Design review of the part built by this model. Coordinates are the model's own, in mm. A direction names the side the tool comes from. Coordinates: 2 decimals unless noted, no trailing zeros. Write each loop counter-clockwise with the first axis right and the second up, starting at its lowest first coordinate (ties: lowest second). Pieces come first, ordered by that corner, then holes.
Q1. Clearance check with flat-ended pins moving along their axes: pin 1 Ø1 at (x, z) = (-9.5, 1.5) entering from -Y; pin 2 Ø8 at (x, y) = (8, 9) entering from -Z; pin 3 Ø3.5 at (x, y) = (0, 6.25) entering from +Z; pin 4 Ø5 at (x, y) = (0, 6.35) entering from -Z. State where each tip first meets the part, or that it passes through.
Q2. Add section A-A, the plane x = 0. Give the boundary of the cut face in (y, z), plus the area to 3 significant figures.
Q3. Add section B-B, the plane z = -9.5. Give the boundary of the cut face in (x, y).
Q4. The part is to be moulded in two halves that separate along X. For faces 1 (the face through (0, 16, 0)), 2 (the face through (-0.9, 7.98, -6.2)), 3 (the face through (-1.009, 9.666, -15.267)), say which applies: +X half, -X half, draft (parallel to the pull), parting line (faces both ways), or undercut.
Q5. To check wall thickness, follow probe 1 along Y at (x, z) = (0, -6.3); probe 2 along X at (y, z) = (7.5, -7); probe 3 along X at (y, z) = (6.35, 12.5). State the ranges of each line that lie inside material, in increasing order.
Q6. Add section C-C, the plane z = 0. Give the boundary of the cut face in (x, y), plus the area to 3 significant figures.
Q7. Machinability: for faces 4 (the face through (-0.931, 3.393, 12.005)), 5 (the face through (-3, 0, 4)), 6 (the face through (0.931, 3.393, -12.005)), 7 (the face through (-4.34, 6.41, 1.8)), which of the approach directions +Z, -Z, +X, -X, +Y, -Y give a long, thin tool a straight path to every point of the face, cutting with its end or side? Answer none if there is none.
Q8. Add section D-D, the plane y = 13.5. Give the boundary of the cut face in (x, z).
Autodesk Inventor part; units mm, degrees
ref_plane "YZ Plane" through (0, 0, 0) normal (1, 0, 0) x (0, 1, 0)
ref_plane "XZ Plane" through (0, 0, 0) normal (0, 1, 0) x (-1, 0, 0)
ref_plane "XY Plane" through (0, 0, 0) normal (0, 0, 1) x (1, 0, 0)
sketch "Sketch1" plane through (0, 0, 0) normal (0, 1, 0) x (-1, 0, 0)
  circle A0 centre (0, 0) radius 15.3
  circle A1 centre (0, 0) radius 4.7
  dimension "d0" = 30.6
  dimension "d1" = 9.4
extrude "Extrusion1" add sketch "Sketch1" along normal blind 13
sketch "Sketch2" plane through (0, 13, 0) normal (0, 1, 0) x (1, 0, 0)
  line L0 (19.8933, 0) -> (-23.0575, 0) construction
  point P0 (0, 0)
ref_plane "Work Plane1" through (19.8933, 13, 0) normal (0, 0, -1) x (-1, 0, 0)
sketch "Sketch3" plane through (19.8933, 13, 0) normal (0, 0, -1) x (-1, 0, 0)
  circle A0 centre (19.8933, -6.75) radius 1.95
  line L0 (35.1933, 0) -> (4.5933, 0)
  line L1 (15.1933, 0) -> (24.5933, 0)
  point P0 (19.8933, -13)
  dimension "d5" = 3.9
  dimension "d18" = 6.75
extrude "Extrusion2" cut sketch "Sketch3" along normal through all both and the other way through all
ref_plane "Work Plane2" through (0, 0, 15.3) normal (0, 0, -1) x (-1, 0, 0)
sketch "Sketch4" plane through (0, 0, 15.3) normal (0, 0, -1) x (-1, 0, 0)
  point P0 (0, 0)
  point P1 (1.95, 6.25)
  point P2 (0, 6.35)
hole "Hole1" at (0, 6.35, 15.3) direction (0, 0, -1) diameter 6.2 depth 6.5 tip angle 118
mirror "Mirror1" about plane through (19.8933, 13, 0) normal (0, 0, -1) of "Hole1"
sketch "Sketch5" plane through (0, 13, 0) normal (0, 1, 0) x (1, 0, 0)
  circle A0 centre (0, 0) radius 15.3
extrude "Extrusion3" add sketch "Sketch5" along normal blind 3
properties part number "brImp_fan"
Here are the results:
1. pin 1: stops at y = 0
1. pin 2: stops at z = -14.77
1. pin 3: passes through
1. pin 4: stops at z = -8.44
2. outline: (0, -15.3) - (3.25, -15.3) - (3.25, -8.8) - (4.3, -8.17) - (4.3, -4.7) - (0, -4.7) - close; (0, 4.7) - (4.3, 4.7) - (4.3, 8.17) - (3.25, 8.8) - (3.25, 15.3) - (0, 15.3) - close; (8.2, -8.05) - (9.45, -8.8) - (9.45, -15.3) - (16, -15.3) - (16, 15.3) - (9.45, 15.3) - (9.45, 8.8) - (8.2, 8.05) - (8.2, 4.7) - (13, 4.7) - (13, -4.7) - (8.2, -4.7) - close
2. area: 253 mm2
3. outline: (-11.99, 0) - (11.99, 0) - (11.99, 16) - (-11.99, 16) - close; hole circle Ø6.2 at (0, 6.35)
4. face 1: draft
4. face 2: undercut
4. face 3: parting line
5. probe 1: y = 0 to 4.3, 8.2 to 16
5. probe 2: x = -13.6 to -1.5, 1.5 to 13.6
5. probe 3: x = -8.82 to -3.1, 3.1 to 8.82
6. outline: (-15.3, 0) - (-4.7, 0) - (-4.7, 13) - (4.7, 13) - (4.7, 0) - (15.3, 0) - (15.3, 16) - (-15.3, 16) - close
6. area: 367 mm2
7. face 4: +Z
7. face 5: +Z, -Z, +X, -X, -Y
7. face 6: -Z
7. face 7: -Y
8. outline: circle Ø30.6 at (0, 0)
